from build123d import *

# Parameters (mm, degrees)
RESSALTO_EXTRUS_O1_DEPTH                            = 98
ESBO_O4_W                                           = 33
ESBO_O4_H                                           = 22
CORTE_EXTRUS_O3_DEPTH                               = 25
ESBO_O2_R                                           = 4
CORTE_EXTRUS_O1_DEPTH                               = 98
ESBO_O10_W                                          = 12
ESBO_O10_H                                          = 4
CORTE_EXTRUS_O8_DEPTH                               = 77
ESBO_O11_R                                          = 1.6
CORTE_EXTRUS_O9_DEPTH                               = 20
ESBO_O12_W                                          = 22
ESBO_O12_H                                          = 40
CORTE_EXTRUS_O10_DEPTH                              = 10
FILETE1_R                                           = 2.5
ESCAREADO_PARA_PARAFUSO_ALLEN_SEXTAVADO_D           = 4.3
ESCAREADO_PARA_PARAFUSO_ALLEN_SEXTAVADO_CSINK_D     = 8.96
ESCAREADO_PARA_PARAFUSO_ALLEN_SEXTAVADO_CSINK_ANGLE = 90
ESBO_O15_W                                          = 4
ESBO_O15_H                                          = 22
CORTE_EXTRUS_O11_DEPTH                              = 13.7


with BuildPart() as part:
    # Esboço1 → Ressalto-extrusão1 (new body)
    with BuildSketch(Plane.XY):
        Polygon((0, 0), (94, 0), (75.862520314, 12.7), (0, 12.7), align=None)
    extrude(amount=RESSALTO_EXTRUS_O1_DEPTH)

    # Esboço4 → Corte-extrusão3 (cut)
    with BuildSketch(Plane(origin=(0, 12.7, 0), x_dir=(1, 0, 0), z_dir=(0, 1, 0))):
        with Locations((16.5, -87)):
            Rectangle(ESBO_O4_W, ESBO_O4_H)
        with Locations((16.5, -11)):
            Rectangle(ESBO_O4_W, ESBO_O4_H)
        with Locations((53.5, -87)):
            Rectangle(ESBO_O4_W, ESBO_O4_H)
        with Locations((53.5, -11)):
            Rectangle(ESBO_O4_W, ESBO_O4_H)
    extrude(amount=-CORTE_EXTRUS_O3_DEPTH, mode=Mode.SUBTRACT)

    # Esboço2 → Corte-extrusão1 (cut)
    with BuildSketch(Plane(origin=(0, 12.7, 0), x_dir=(1, 0, 0), z_dir=(0, 1, 0))):
        with Locations((76, -92)):
            Circle(ESBO_O2_R)
        with Locations((76, -6)):
            Circle(ESBO_O2_R)
        with Locations((5, -49)):
            Circle(ESBO_O2_R)
    extrude(amount=-CORTE_EXTRUS_O1_DEPTH, mode=Mode.SUBTRACT)

    # Esboço10 → Corte-extrusão8 (cut, through all)
    with BuildSketch(Plane.XY.offset(76)):
        with Locations((16.5, 10.7)):
            Rectangle(ESBO_O10_W, ESBO_O10_H)
        with Locations((53.5, 10.7)):
            Rectangle(ESBO_O10_W, ESBO_O10_H)
    extrude(amount=-CORTE_EXTRUS_O8_DEPTH, mode=Mode.SUBTRACT)

    # Esboço11 → Corte-extrusão9 (cut)
    with BuildSketch(Plane(origin=(0, 12.7, 0), x_dir=(1, 0, 0), z_dir=(0, 1, 0))):
        with Locations((29.25, -26.5)):
            Circle(ESBO_O11_R)
        with Locations((29.25, -71.5)):
            Circle(ESBO_O11_R)
        with Locations((3.75, -71.5)):
            Circle(ESBO_O11_R)
        with Locations((3.75, -26.5)):
            Circle(ESBO_O11_R)
        with Locations((40.75, -26.5)):
            Circle(ESBO_O11_R)
        with Locations((66.25, -26.5)):
            Circle(ESBO_O11_R)
        with Locations((66.25, -71.5)):
            Circle(ESBO_O11_R)
        with Locations((40.75, -71.5)):
            Circle(ESBO_O11_R)
    extrude(amount=-CORTE_EXTRUS_O9_DEPTH, mode=Mode.SUBTRACT)

    # Esboço12 → Corte-extrusão10 (cut)
    with BuildSketch(Plane(origin=(0, 12.7, 0), x_dir=(1, 0, 0), z_dir=(0, 1, 0))):
        with Locations((35, -49)):
            Rectangle(ESBO_O12_W, ESBO_O12_H)
    extrude(amount=-CORTE_EXTRUS_O10_DEPTH, mode=Mode.SUBTRACT)

    # Filete1
    filete1_edges = [part.edges().sort_by_distance(p)[0] for p in [
        (46, 7.7, 29),
        (46, 7.7, 69),
        (24, 7.7, 69),
        (24, 7.7, 29),
    ]]
    fillet(filete1_edges, radius=FILETE1_R)

    # Escareado para parafuso Allen sextavado escareado de M41 (through all)
    with Locations(Plane(origin=(0, 0, 0), x_dir=(-1, 0, 0), z_dir=(0, -1, 0))):
        with Locations((-66.25, -71.5), (-66.25, -26.5), (-40.75, -26.5), (-29.25, -26.5), (-29.25, -71.5), (-40.75, -71.5), (-3.75, -71.5), (-3.75, -26.5)):
            CounterSinkHole(ESCAREADO_PARA_PARAFUSO_ALLEN_SEXTAVADO_D / 2, ESCAREADO_PARA_PARAFUSO_ALLEN_SEXTAVADO_CSINK_D / 2, counter_sink_angle=ESCAREADO_PARA_PARAFUSO_ALLEN_SEXTAVADO_CSINK_ANGLE)

    # Esboço15 → Corte-extrusão11 (cut, through all)
    with BuildSketch(Plane(origin=(0, 12.7, 0), x_dir=(1, 0, 0), z_dir=(0, 1, 0))):
        with Locations((35, -11)):
            Rectangle(ESBO_O15_W, ESBO_O15_H)
        with Locations((35, -87)):
            Rectangle(ESBO_O15_W, ESBO_O15_H)
    extrude(amount=-CORTE_EXTRUS_O11_DEPTH, mode=Mode.SUBTRACT)


solid = part.part
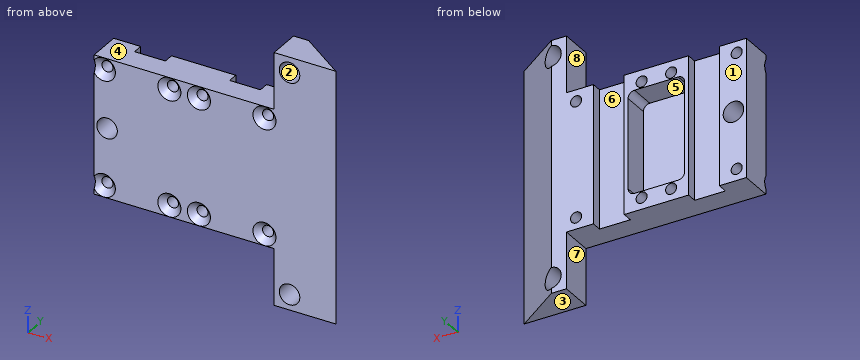
Geometry: final body of the model. Coordinates: model frame, mm. Face numbers are marked on the shaded views. A direction names the side the tool comes from. Give positions to 0.01 mm unless a question says otherwise; leave off trailing zeros. Loops run counter-clockwise (first coordinate to the right, second up) from the corner with the lowest first, then second, coordinate; pieces in that order, holes last. Notation, with made-up numbers: M 48,0 L 53,0 A20 ccw 53,30 Z; hole C 28,27 d11. An arc over 180 degrees is marked long. Put each result on its own line as item: value. Start each with the question number.
1) Ray query, line 1 along Z through (x, y) = (66.25, 8); line 2 along Z through (x, y) = (76, 8.5); line 3 along Z through (x, y) = (29.25, 5.5). Return the intervals inside material, ascending.
2) Access query for the marked faces 5, 6, 7 and 8. Directions: +Z, -Z, +X, -X, +Y, -Y. A direction counts if a zero-diameter tool reaches every point of the face in a straight line with its end or side. Return the directions, or none.
3) Contact query for flat-ended pins moving along their axis: pin 1 (1 mm diameter, centred on x = 64, y = 10.5, fed in from -Z); pin 2 (4 mm diameter, centred on y = 8, z = 6, fed in from -X); pin 3 (5 mm diameter, centred on y = 10.5, z = 82, fed in from +X). Output: stop coordinate, or through.
4) Cut plane B-B (z = 49). Output: boundary loops of the cut face in (x, y).
5) Pull-direction query (Z, two-part tool) for the marked faces 1, 2, 3 and 4; classes: pulls with the +Z half, pulls with the -Z half, needs draft (parallel to the pull), parting line crosses it, or undercut.
6) Cut plane A-A (x = 66.25). Give the number of separate pieces and of enclosed holes in the cut face, then the cut area to 3 significant figures.
7) Cut plane D-D (z = 35). Output: boundary loops of the cut face in (x, y), then the cut area to 3 significant figures.
Verdict:
1. line 1: 22 to 24.35, 28.65 to 69.35, 73.65 to 76
1. line 2: 0 to 2, 10 to 88, 96 to 98
1. line 3: 22 to 24.35, 28.65 to 29, 69 to 69.35, 73.65 to 76
2. face 5: +Y
2. face 6: +Z, -Z, +Y
2. face 7: -Z, -X, +Y, -Y
2. face 8: +Z, -X, +Y, -Y
3. pin 1: z = 22
3. pin 2: x = 70
3. pin 3: x = 82.57
4. outline: M 0,0 L 1,0 L 1,12.7 L 0,12.7 Z; M 9,0 L 94,0 L 75.86,12.7 L 59.5,12.7 L 59.5,8.7 L 47.5,8.7 L 47.5,12.7 L 46,12.7 L 46,2.7 L 24,2.7 L 24,12.7 L 22.5,12.7 L 22.5,8.7 L 10.5,8.7 L 10.5,12.7 L 9,12.7 Z
5. face 1: needs draft
5. face 2: undercut
5. face 3: pulls with the -Z half
5. face 4: pulls with the +Z half
6. separate pieces: 3
6. enclosed holes: 0
6. area: 566 mm2
7. outline: M 0,0 L 94,0 L 75.86,12.7 L 59.5,12.7 L 59.5,8.7 L 47.5,8.7 L 47.5,12.7 L 46,12.7 L 46,2.7 L 24,2.7 L 24,12.7 L 22.5,12.7 L 22.5,8.7 L 10.5,8.7 L 10.5,12.7 L 0,12.7 Z
7. area: 763 mm2
